The listing builds one solid part. Answer for the finished solid, in the listing's coordinates (mm). A direction names the side the tool comes from. Give positions to 0.01 mm unless a question says otherwise; leave off trailing zeros. Order: outer loops, then holes, each group sorted by start corner. A loop starts at its lowest first (then second) coordinate and runs counter-clockwise, first axis right, second up. Notation, with made-up numbers: (68.25, 69.25) - (112.25, 69.25) arc R33 ccw to (112.25, 101.25) - close; hole circle Ø5 at (58.5, -33). An arc over 180 degrees is marked (long way). Answer in a Markdown table with one row per item. Add a question column.
Autodesk Inventor part; units mm, degrees
ref_plane "YZ Plane" through (0, 0, 0) normal (1, 0, 0) x (0, 1, 0)
ref_plane "XZ Plane" through (0, 0, 0) normal (0, 1, 0) x (-1, 0, 0)
ref_plane "XY Plane" through (0, 0, 0) normal (0, 0, 1) x (1, 0, 0)
sketch "Sketch1" plane through (0, 0, 0) normal (0, 0, 1) x (1, 0, 0)
  line L0 (0, 0) -> (7.6, 0)
  line L1 (12, -2.5403) -> (12, -6.4)
  line L2 (12, -6.4) -> (5, -6.4)
  line L3 (5, -6.4) -> (5, -16.4)
  line L4 (5, -16.4) -> (0, -16.4)
  line L5 (0, -16.4) -> (0, 0)
  line L6 (7.6, 0) -> (12, -2.5403)
  dimension "d0" = 24
  dimension "d1" = 10
  dimension "d2" = 6.4
  dimension "d3" = 10
  dimension "d20" = 30
  dimension "d21" = 15.2
revolve "Вращение1" add sketch "Sketch1" angle 360 about axis through (0, -16.4, 0) along (0, 1, 0)
sketch "Sketch2" plane through (0, 0, 0) normal (0, 1, 0) x (1, 0, 0)
  line L0 (0, -9.2376) -> (-8, -4.6188)
  line L1 (-8, -4.6188) -> (-8, 4.6188)
  line L2 (-8, 4.6188) -> (0, 9.2376)
  line L3 (0, 9.2376) -> (8, 4.6188)
  line L4 (8, 4.6188) -> (8, -4.6188)
  line L5 (8, -4.6188) -> (0, -9.2376)
  circle A0 centre (0, 0) radius 12
  point P0 (0, 0)
  point P1 (0, 0)
  dimension "d22" = 16
extrude "Выдавливание1" cut sketch "Sketch2" against normal blind 6.4
thread "Резьба1"
chamfer "Фаска1" distance 0.8333 angle 45 1 edges at (-5, -16.4, 0)
equation "\"d22\" = S_"
equation "\"d23\" = k"
equation "\"d12\" = b"
equation "\"d14\" = 0.0833333 * d"
equation "\"d0\" = 1.5 * S_"
equation "\"d1\" = d1_"
equation "\"d2\" = k"
equation "\"d3\" = L"
equation "\"d21\" = 0.95 * S_"
equation "\"d1_\" = 10"
equation "\"S_\" = 16"
equation "\"k\" = 6.4"
equation "\"e\" = 17.6"
equation "\"L\" = 10"
equation "\"b\" = 8"
equation "\"Grip_Length\" = 2"
properties part number "Болт M10-6g×10(S16) ГОСТ 7798-70" material "Сталь, мягкая"
(1) Find section B-B, the plane y = -14.75. Write down the section's boundary in (x, z).
(2) For faces 1 (the face through (-1.08, -11.05, -4.88)), 2 (the face through (0, 0, 0)), determine the directions among +Z, -Z, +X, -X, +Y, -Y from which every point of the face is accessible in a straight line to the end or side of a thin tool.
(3) Each of these flat-tipped pins is pushed along its axis until it touches: P1, Ø8, axis at y = -3.5, z = 6, coming from the -X side; P2, Ø2, axis at x = -4, y = -3.5, coming from the -Z side; P3, Ø5, axis at x = 1.5, y = -13, coming from the -Z side; P4, Ø4, axis at x = 1.5, y = -8, coming from the +Z side. Where does it stop, or does it pass through?
(4) Straight lines are drawn through the part: line 1 (Y direction, x = -6, z = 4.25); line 2 (X direction, y = -2, z = 6.5); line 3 (X direction, y = -3.75, z = 5.25). For each, find the intervals that lie inside material, in ascending order.
(5) Find section A-A, the plane z = 0. Write down the section's boundary in (x, y).
Answer key:
| question | item | result |
|---|---|---|
| 1 | outline | circle Ø10 at (0, 0) |
| 2 | face 1 | -Y |
| 2 | face 2 | +Z, -Z, +X, -X, +Y |
| 3 | P1 | x = -8 |
| 3 | P2 | z = -7.51 |
| 3 | P3 | z = -5 |
| 3 | P4 | z = 9.06 |
| 4 | line 1 | -6.4 to 0 |
| 4 | line 2 | -4.74 to 4.74 |
| 4 | line 3 | -6.91 to 6.91 |
| 5 | outline | (-8, -6.4) - (-5, -6.4) - (-5, -15.57) - (-4.17, -16.4) - (4.17, -16.4) - (5, -15.57) - (5, -6.4) - (8, -6.4) - (8, -0.23) - (7.6, 0) - (-7.6, 0) - (-8, -0.23) - close |
